Geometry check sheet. Reference: the model listing, model coordinates, mm. A direction names the side the tool comes from. Round coordinates to 2 decimals unless told otherwise and drop trailing zeros. Loops run counter-clockwise (first coordinate to the right, second up) from the corner with the lowest first, then second, coordinate; pieces in that order, holes last. Notation, with made-up numbers: (74, 44.25) -> (109, 44.25) arc R11 ccw to (109, 62.25) -> close; hole circle Ø8 at (-31, 70.5). An arc over 180 degrees is marked (long way). Use a Markdown table: item, result. Add a question column.
Q1. Gauge pin test, flat ends, axial feed: P1, Ø3, axis at y = -42.5, z = 1, coming from the +X side; P2, Ø1.6, axis at x = -12, z = -15.5, coming from the -Y side; P3, Ø3, axis at x = -13, y = -47, coming from the -Z side. Record the tip position at first contact, or that the pin passes through.
Q2. Material ranges on L1, parallel to Z at x = -89.5, y = -30.5; L2, parallel to Z at x = -47, y = -15; L3, parallel to Y at x = -62.5, z = -1.75, recorded low to high.
Q3. Sectioned sample at B-B, the plane y = -30. Enter the section's corners in (x, z).
Q4. Sectioned sample at A-A, the plane x = -40. Enter the section's corners in (y, z).
Q5. Sectioned sample at D-D, the plane z = -9.75. Enter the section's corners in (x, y).
Q6. Sectioned sample at C-C, the plane x = 71. Enter the section's corners in (y, z), then the cut area to 3 significant figures.
Q7. Set-up check for faces 1 (the face through (-11, -44, 0)), 2 (the face through (-8, -5.028, -7)): record each of +Z, -Z, +X, -X, +Y, -Y from which the full face is reachable in a straight line by a thin tool's end or side.
```python
from build123d import *

# Parameters (mm, degrees)
F1_DEPTH = 3
F2_W     = 200
F2_H     = 17
F3_DEPTH = 3
F4_R     = 15


with BuildPart() as f1:
    # F0 (on Top) → F1 (new body)
    with BuildSketch(Plane.XY):
        with BuildLine():
            Line((91.016510874, -5.0278047089), (-108.983489126, -5.0278047089))
            Line((-108.983489126, -5.0278047089), (-108.983489126, -65.0278047089))
            Line((-108.983489126, -65.0278047089), (41.016510874, -65.0278047089))
            ThreePointArc((41.016510874, -65.0278047089), (76.3718499334, -50.3831437682), (91.016510874, -15.0278047089))
            Line((91.016510874, -15.0278047089), (91.016510874, -5.0278047089))
        make_face()
    extrude(amount=F1_DEPTH)

    # F2 (on face) → F3 (join)
    with BuildSketch(Plane(origin=(0, -5.0278047089, 0), x_dir=(-1, 0, 0), z_dir=(0, 1, 0))):
        with Locations((8.983489126, -8.5)):
            Rectangle(F2_W, F2_H)
    extrude(amount=-F3_DEPTH)

    # F4
    f4_edges = [f1.edges().sort_by_distance(p)[0] for p in [
        (-8.983489, -8.027805, 0),
    ]]
    fillet(f4_edges, radius=F4_R)


solid = f1.part
```
Values:
| question | item | result |
|---|---|---|
| 1 | P1 | x = 83.74 |
| 1 | P2 | y = -8.03 |
| 1 | P3 | z = 0 |
| 2 | L1 | 0 to 3 |
| 2 | L2 | -2.33 to 3 |
| 2 | L3 | -16 to -5.03 |
| 3 | outline | (-108.98, 0) -> (88.72, 0) -> (88.72, 3) -> (-108.98, 3) -> close |
| 4 | outline | (-65.03, 0) -> (-23.03, 0) arc R15 cw to (-8.03, -15) -> (-8.03, -17) -> (-5.03, -17) -> (-5.03, 3) -> (-65.03, 3) -> close |
| 5 | outline | (-108.98, -8.98) -> (91.02, -8.98) -> (91.02, -5.03) -> (-108.98, -5.03) -> close |
| 6 | outline | (-55.04, 0) -> (-23.03, 0) arc R15 cw to (-8.03, -15) -> (-8.03, -17) -> (-5.03, -17) -> (-5.03, 3) -> (-55.04, 3) -> close |
| 6 | area | 249 mm^2 |
| 7 | face 1 | -Z, +X, -X, -Y |
| 7 | face 2 | +Z, -Z, +X, -X, +Y |
